```python
from build123d import *

# Parameters (mm, degrees)
SKETCH_1_W      = 130
SKETCH_1_H      = 30
EXTRUDE_1_DEPTH = 25
SKETCH_2_R      = 4
EXTRUDE_2_DEPTH = 5


with BuildPart() as part:
    # 草图1 → 凸台-拉伸1 (new body)
    with BuildSketch(Plane(origin=(0, 0, 0), x_dir=(1, 0, 0), z_dir=(0, 1, 0))):
        Rectangle(SKETCH_1_W, SKETCH_1_H)
    extrude(amount=EXTRUDE_1_DEPTH)

    # 草图2 → 凸台-拉伸2 (add)
    with BuildSketch(Plane.ZY.offset(65)):
        with Locations(Location((-8, 12.5, 0), (0, 0, 180))):
            Circle(SKETCH_2_R)
        with Locations(Location((8, 12.5, 0), (0, 0, 180))):
            Circle(SKETCH_2_R)
    extrude(amount=EXTRUDE_2_DEPTH)


solid = part.part
```
Model file for the job. Use its own axes, mm. A direction names the side the tool comes from. Give positions to 0.01 mm unless a question says otherwise; leave off trailing zeros. Loops run counter-clockwise (first coordinate to the right, second up) from the corner with the lowest first, then second, coordinate; pieces in that order, holes last. Notation, with made-up numbers: (60, 62) - (116, 62) arc R18 ccw to (116, 77) - close; hole circle Ø9 at (-11, 84.5). An arc over 180 degrees is marked (long way). One line per item, written item: value. Start each with the question number.
1. Which spindle directions (+Z, -Z, +X, -X, +Y, -Y) get a long thin tool onto all of the face, cutting with end or side? Do faces 1 (the flat face through (-70, 12, -8)), 2 (the cylindrical face through (-67.5, 14.9, -4.8)). Say none if no direction does.
2. Pull direction Z, two halves, no side cores. Call faces 3 (the cylindrical face through (-67.5, 14.9, 11.2)), 4 (the flat face through (-1, 12, 15)), 5 (the flat face through (65, 12, 0)): pulls with the +Z half, pulls with the -Z half, needs draft (parallel to the pull), parting line crosses it, or undercut.
3. Slice it at D-D (y = 3). List the corners of the cut face in (x, z).
4. Probe L1, parallel to X at y = 7.25, z = 0.25. List the from-to ranges inside material, lowest first. Write a range as from..to.
5. Slice it at A-A (z = 8). List the corners of the cut face in (x, y).
6. Slice it at B-B (y = 12.5). List the corners of the cut face in (x, z).
7. Slice it at C-C (z = -5.5). List the corners of the cut face in (x, y).
Solution:
1. face 1: +Z, -Z, -X, +Y, -Y
1. face 2: -X
2. face 3: undercut
2. face 4: pulls with the +Z half
2. face 5: needs draft
3. outline: (-65, -15) - (65, -15) - (65, 15) - (-65, 15) - close
4. L1: x = -65..65
5. outline: (-70, 8.5) - (-65, 8.5) - (-65, 0) - (65, 0) - (65, 25) - (-65, 25) - (-65, 16.5) - (-70, 16.5) - close
6. outline: (-70, -12) - (-65, -12) - (-65, -15) - (65, -15) - (65, 15) - (-65, 15) - (-65, 12) - (-70, 12) - (-70, 4) - (-65, 4) - (-65, -4) - (-70, -4) - close
7. outline: (-70, 9.38) - (-65, 9.38) - (-65, 0) - (65, 0) - (65, 25) - (-65, 25) - (-65, 15.62) - (-70, 15.62) - close
